Could you check a few things on this model? Use its own coordinates, in mm. Face numbers are marked on the shaded views. A direction names the side the tool comes from. Coordinates: 2 decimals unless noted, no trailing zeros. Order: outer loops, then holes, each group sorted by start corner. A loop starts at its lowest first (then second) coordinate and runs counter-clockwise, first axis right, second up. Notation, with made-up numbers: (89, 12.5) - (93, 12.5) arc R8 ccw to (93, 17.5) - close; hole circle Ø9 at (55.25, -25). An arc over 180 degrees is marked (long way). One line per item, written item: value.
from build123d import *


with BuildPart() as part:
    # Sketch1 → Revolve-Thin1 (revolve)
    with BuildSketch(Plane(origin=(0, 0, 0), x_dir=(0, 0, -1), z_dir=(1, 0, 0)), mode=Mode.PRIVATE) as revolve_thin1_sk:
        with BuildLine():
            Line((0, 0.9), (4.471714314, 0.9))
            ThreePointArc((4.471714314, 0.9), (4.859012649, 0.978045554), (5.185857157, 1.2))
            ThreePointArc((5.185857157, 1.2), (5.512701665, 1.421954446), (5.9, 1.5))
            Line((5.9, 1.5), (10.4, 1.5))
            Line((10.4, 1.5), (10.4, 1.6))
            Line((10.4, 1.6), (5.9, 1.6))
            ThreePointArc((5.9, 1.6), (5.473971832, 1.51414989), (5.114442873, 1.27))
            ThreePointArc((5.114442873, 1.27), (4.820282815, 1.070240999), (4.471714314, 1))
            Line((4.471714314, 1), (0, 1))
            Line((0, 1), (0, 0.9))
        make_face()
    revolve(revolve_thin1_sk.sketch.rotate(Axis((0, 0, 0), (0, 0, -1)), 90), axis=Axis((0, 0, 0), (0, 0, -1)))


solid = part.part
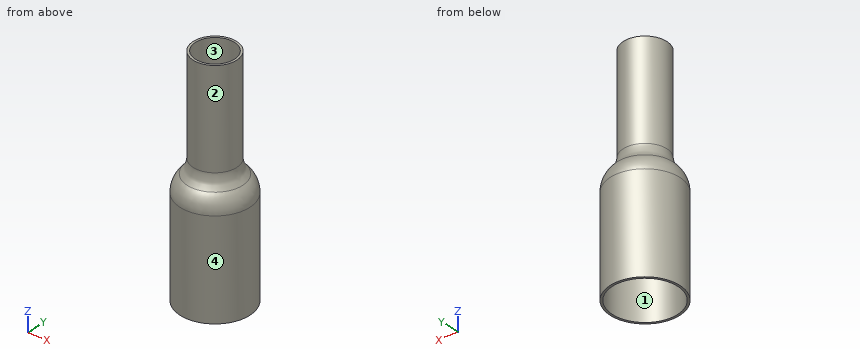
Item 1: For the marked faces 1 and 2, which set-ups out of +Z, -Z, +X, -X, +Y, -Y let a thin tool reach every point of the face, with its end or its side?
Conclusion:
face 1: -Z
face 2: +Z
Item 2: If I drill on probe 1 along Z at (x, y) = (0.35, -1.3); probe 2 along Z at (x, y) = (-1.3, -0.3), over which ranges is the centre line in solid material (lowest first)?
Conclusion:
probe 1: -5.37 to -5.2
probe 2: -5.35 to -5.18
Item 3: I want a section at B-B on z = -4.25. Please give me the cut outline in (x, y).
Conclusion:
outline: circle Ø2 at (0, 0); hole circle Ø1.8 at (0, 0)
Item 4: I'm going to push a flat-ended pin straight in: pin 1 Ø1 at (x, z) = (0, -4) entering from +Y. Where does the tip first touch, or does it pass through?
Conclusion:
pin 1: y = 1
Item 5: Thinking about a two-plate mould opening in Y: for the marked faces 3 and 4, which applies, pulls with the +Y half, pulls with the -Y half, needs draft (parallel to the pull), parting line crosses it, or undercut?
Conclusion:
face 3: undercut
face 4: parting line crosses it
Item 6: I want a section at A-A on z = -7.25. Please give me the cut outline in (x, y).
Conclusion:
outline: circle Ø3.2 at (0, 0); hole circle Ø3 at (0, 0)
